```python
from build123d import *

# Parameters (mm, degrees)
SKETCH_W     = 150
SKETCH_H     = 150
SKETCH_W_2   = 110
SKETCH_H_2   = 110
PAD_DEPTH    = 10
SKETCH003_W  = 20
SKETCH003_H  = 20
PAD001_DEPTH = 10


with BuildPart() as part:
    # Sketch → Pad (new body)
    with BuildSketch(Plane.XY):
        Rectangle(SKETCH_W, SKETCH_H)
        Rectangle(SKETCH_W_2, SKETCH_H_2, mode=Mode.SUBTRACT)
    extrude(amount=PAD_DEPTH)

    # Sketch003 → Pad001 (new body)
    with BuildSketch(Plane(origin=(0, 0, 0), x_dir=(1, 0, 0), z_dir=(0, 0, -1))):
        with Locations((-65, 0)):
            Rectangle(SKETCH003_W, SKETCH003_H)
    extrude(amount=PAD001_DEPTH)


solid = part.part
```
Part model, mm, in its own coordinate system. A direction names the side the tool comes from. Round coordinates to 2 decimals unless told otherwise and drop trailing zeros. Write each loop counter-clockwise with the first axis right and the second up, starting at its lowest first coordinate (ties: lowest second). Pieces come first, ordered by that corner, then holes. Notation, with made-up numbers: (-6, -9) -> (8, -9) arc R16 ccw to (8, -4) -> close; hole circle Ø8 at (85.5, 62). An arc over 180 degrees is marked (long way). Return JSON: item names as keys, results as strings. Group by question number.
Q1. Saw through at A-A on y = 2. Write the cut outline in (x, z).
Q2. Saw through at D-D on z = -5.25. Write the cut outline in (x, y), plus the area to 3 significant figures.
Q3. Which spindle directions (+Z, -Z, +X, -X, +Y, -Y) get a long thin tool onto all of the face, cutting with end or side? Do faces 5 (the flat face through (-65, 10, -5)), 6 (the flat face through (-55, -1, 4)), 7 (the flat face through (-65, -10, -5)). Say none if no direction does.
Q4. Pin check, flat tips, straight feed: pin 1 (8 mm diameter, centred on x = -64.5, z = -7, fed in from +Y); pin 2 (8 mm diameter, centred on x = -41, y = -58, fed in from -Z). Stop position of each tip, or through.
Q5. Probe L1, parallel to Y at x = 26, z = 3.25; L2, parallel to Y at x = -58, z = -5. List the from-to ranges inside material, lowest first. Write a range as [from, to].
Q6. Saw through at B-B on x = 20. Write the cut outline in (y, z).
Q7. Mould opens along X. For faces 1 (the flat face through (55, -1, 5)), 2 (the flat face through (-75, -1, 4)), 3 (the flat face through (-1, -55, 5)), 4 (the flat face through (-68, 1, 10)) say: pulls with the +X half, pulls with the -X half, needs draft (parallel to the pull), parting line crosses it, or undercut.
Q8. Saw through at C-C on x = -57. Write the cut outline in (y, z), plus the area to 3 significant figures.
Answer:
{
 "1": {"outline": "(-75, -10) -> (-55, -10) -> (-55, 10) -> (-75, 10) -> close; (55, 0) -> (75, 0) -> (75, 10) -> (55, 10) -> close"},
 "2": {"outline": "(-75, -10) -> (-55, -10) -> (-55, 10) -> (-75, 10) -> close", "area": "400 mm2"},
 "3": {"face 5": "-Z, +X, -X, +Y", "face 6": "+Z, -Z", "face 7": "-Z, +X, -X, -Y"},
 "4": {"pin 1": "y = 10", "pin 2": "z = 0"},
 "5": {"L1": "[-75, -55], [55, 75]", "L2": "[-10, 10]"},
 "6": {"outline": "(-75, 0) -> (-55, 0) -> (-55, 10) -> (-75, 10) -> close; (55, 0) -> (75, 0) -> (75, 10) -> (55, 10) -> close"},
 "7": {"face 1": "undercut", "face 2": "pulls with the -X half", "face 3": "undercut", "face 4": "needs draft"},
 "8": {"outline": "(-75, 0) -> (-10, 0) -> (-10, -10) -> (10, -10) -> (10, 0) -> (75, 0) -> (75, 10) -> (-75, 10) -> close", "area": "1,700 mm2"}
}
